from build123d import *

# Parameters (mm, degrees)
F1_DEPTH = 25.4
F2_R     = 12.7
F3_R     = 12.69999
F4_R     = 12.7
F5_R     = 12.69999
F7_DEPTH = 25.4
F8_R     = 6.35
F9_DEPTH = 31.75


# Not quite as in the source:
# - a fillet or chamfer is up to 0.001 mm smaller than in the source, because OpenCascade refuses the exact size


with BuildPart() as f1:
    # F0 (on Front) → F1 (new body)
    with BuildSketch(Plane.XZ):
        Polygon((0, 38.1), (0, 0), (63.5, 0), (63.5, 12.7), (25.4, 12.7), (25.4, 38.1), align=None)
    extrude(amount=F1_DEPTH)

    # F2
    f2_edges = [f1.edges().sort_by_distance(p)[0] for p in [
        (63.5, -25.4, 6.35),
    ]]
    fillet(f2_edges, radius=F2_R)

    # F3 (radius 12.7 in the source; OpenCascade refuses exactly that, so slightly less here)
    f3_edges = [f1.edges().sort_by_distance(p)[0] for p in [
        (63.5, 0, 6.35),
    ]]
    fillet(f3_edges, radius=F3_R)

    # F4
    f4_edges = [f1.edges().sort_by_distance(p)[0] for p in [
        (25.4, -12.7, 38.1),
    ]]
    fillet(f4_edges, radius=F4_R)

    # F5 (radius 12.7 in the source; OpenCascade refuses exactly that, so slightly less here)
    f5_edges = [f1.edges().sort_by_distance(p)[0] for p in [
        (0, -12.7, 38.1),
    ]]
    fillet(f5_edges, radius=F5_R)

    # F6 (on face) → F7 (cut)
    with BuildSketch(Plane.XY.offset(12.7)):
        with BuildLine():
            ThreePointArc((38.3966746256, -19.0430658334), (42.6938210606, -17.0839831277), (44.45, -12.7))
            ThreePointArc((44.45, -12.7), (42.5901280605, -8.2098719395), (38.1, -6.35))
            ThreePointArc((38.1, -6.35), (31.7518177342, -12.5480726474), (37.7962322754, -19.0427301038))
            Line((37.7962322754, -19.0427301038), (38.3966746256, -19.0430658334))
        make_face()
        with BuildLine():
            ThreePointArc((50.79644948, -19.0499990074), (46.3086168165, -17.1888725866), (44.45, -12.7))
            ThreePointArc((44.45, -12.7), (42.6938210606, -17.0839831277), (38.3966746256, -19.0430658334))
            Line((38.3966746256, -19.0430658334), (50.79644948, -19.0499990074))
        make_face()
        with BuildLine():
            ThreePointArc((38.1, -6.35), (42.5901280605, -8.2098719395), (44.45, -12.7))
            ThreePointArc((44.45, -12.7), (46.3098719395, -8.2098719395), (50.8, -6.35))
            Line((50.8, -6.35), (38.1, -6.35))
        make_face()
        with BuildLine():
            ThreePointArc((50.8, -6.35), (46.3098719395, -8.2098719395), (44.45, -12.7))
            ThreePointArc((44.45, -12.7), (46.3086168165, -17.1888725866), (50.79644948, -19.0499990074))
            ThreePointArc((50.79644948, -19.0499990074), (55.2888725866, -17.1913831835), (57.15, -12.7))
            ThreePointArc((57.15, -12.7), (55.2901280605, -8.2098719395), (50.8, -6.35))
        make_face()
        with BuildLine():
            ThreePointArc((37.7962322754, -19.0427301038), (38.09644948, -19.0499990074), (38.3966746256, -19.0430658334))
            Line((38.3966746256, -19.0430658334), (37.7962322754, -19.0427301038))
        make_face()
    extrude(amount=-F7_DEPTH, mode=Mode.SUBTRACT)

    # F8 (on face) → F9 (cut)
    with BuildSketch(Plane.XZ.offset(25.4)):
        with Locations((12.7, 25.4)):
            Circle(F8_R)
    extrude(amount=-F9_DEPTH, mode=Mode.SUBTRACT)


solid = f1.part
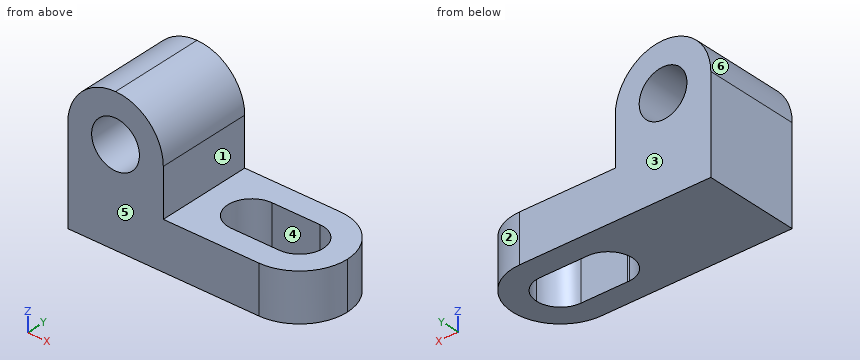
CAD build for the part. Positions are in the model's coordinates, mm. Face numbers are marked on the shaded views. A direction names the side the tool comes from. Give positions to 0.01 mm unless a question says otherwise; leave off trailing zeros. Loops run counter-clockwise (first coordinate to the right, second up) from the corner with the lowest first, then second, coordinate; pieces in that order, holes last. Notation, with made-up numbers: M 28.5,77 L 42.5,77 A22 ccw 42.5,98 Z; hole C -36.5,-2 d6. An arc over 180 degrees is marked long. One line per question, with ' | ' between items. Start each with the question number.
1. Flat gauge pins, fed straight in: pin 1 (1.5 mm diameter, centred on y = -18, z = 16.5, fed in from +X); pin 2 (11.5 mm diameter, centred on x = 12.7, z = 25.4, fed in from +Y); pin 3 (7.5 mm diameter, centred on x = 36, y = -16, fed in from +Z). Where does each tip first touch, or does it go through?
2. Probe L1, parallel to X at y = -1.75, z = 25; L2, parallel to X at y = -12.5, z = 11; L3, parallel to Z at x = 38, y = -21.5. List the from-to ranges inside material, lowest first. Write a range as from..to.
3. Two-plate mould, pull along Y, no slides. Class the marked faces 3, 4, 5 and 6: pulls with the +Y half, pulls with the -Y half, needs draft (parallel to the pull), parting line crosses it, or undercut.
4. Saw through at A-A on y = -12. State how many separate pieces and enclosed holes the cut face has, plus the area to 3 significant figures.
5. 3-axis set-ups, long thin cutter, end or side, ignore diameter. For the marked faces 1 and 2: which of +Z, -Z, +X, -X, +Y, -Y reach the whole face in a straight line?
6. Saw through at C-C on z = 24. Give the cut face in (x, y).
Result sheet:
1) pin 1: stops at x = 25.4 | pin 2: passes through | pin 3: stops at z = 12.7
2) L1: x = 0..6.36, 19.04..25.4 | L2: x = 0..31.75, 57.15..63.5 | L3: z = 0..12.7
3) face 3: pulls with the +Y half | face 4: undercut | face 5: pulls with the -Y half | face 6: needs draft
4) separate pieces: 2 | enclosed holes: 1 | area: 934 mm^2
5) face 1: +Z, +X, +Y, -Y | face 2: +Z, -Z, +X, +Y
6) outline: M 0,-25.4 L 6.51,-25.4 L 6.51,0 L 0,0 Z; M 18.89,-25.4 L 25.4,-25.4 L 25.4,0 L 18.89,0 Z
